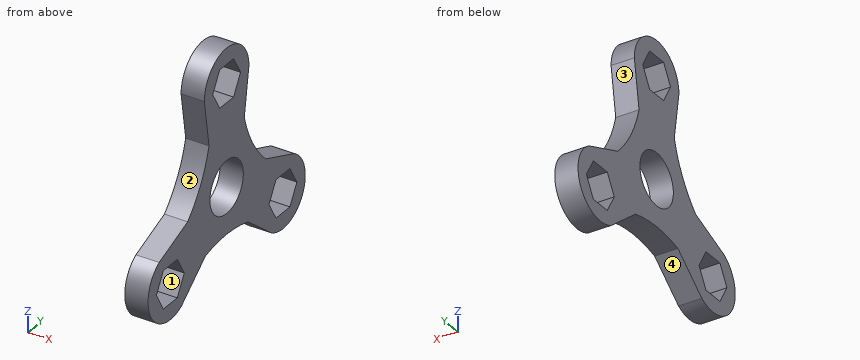
```python
from build123d import *

# Parameters (mm, degrees)
F0_R     = 9
F1_DEPTH = 8


with BuildPart() as f1:
    # F0 (on Right) → F1 (new body)
    with BuildSketch(Plane.YZ):
        with BuildLine():
            Line((9.482996, 18.707991), (12, 35))
            ThreePointArc((12, 35), (0, 47), (-12, 35))
            Line((-12, 35), (-9.482996, 18.707991))
            ThreePointArc((-9.482996, 18.707991), (-13.851316, 7.997061), (-20.943094, -1.14148))
            Line((-20.943094, -1.14148), (-36.310889, -7.107695))
            ThreePointArc((-36.310889, -7.107695), (-40.703194, -23.5), (-24.310889, -27.892305))
            Line((-24.310889, -27.892305), (-11.460098, -17.566512))
            ThreePointArc((-11.460098, -17.566512), (0, -15.994123), (11.460098, -17.566512))
            Line((11.460098, -17.566512), (24.310889, -27.892305))
            ThreePointArc((24.310889, -27.892305), (40.703194, -23.5), (36.310889, -7.107695))
            Line((36.310889, -7.107695), (20.943094, -1.14148))
            ThreePointArc((20.943094, -1.14148), (13.851316, 7.997061), (9.482996, 18.707991))
        make_face()
        Polygon((-26.558112, -11), (-22.805336, -17.5), (-26.558112, -24), (-34.063666, -24), (-37.816443, -17.5), (-34.063666, -11), align=None, mode=Mode.SUBTRACT)
        Polygon((22.805336, -17.5), (26.558112, -11), (34.063666, -11), (37.816443, -17.5), (34.063666, -24), (26.558112, -24), align=None, mode=Mode.SUBTRACT)
        Circle(F0_R, mode=Mode.SUBTRACT)
        Polygon((7.505553, 35), (3.752777, 28.5), (-3.752777, 28.5), (-7.505553, 35), (-3.752777, 41.5), (3.752777, 41.5), align=None, mode=Mode.SUBTRACT)
    extrude(amount=F1_DEPTH)


solid = f1.part
```
Work out the finished part from the listing and answer in its coordinate system (mm). Face numbers are marked on the shaded views. A direction names the side the tool comes from. Give positions to 0.01 mm unless a question says otherwise; leave off trailing zeros. Loops run counter-clockwise (first coordinate to the right, second up) from the corner with the lowest first, then second, coordinate; pieces in that order, holes last. Notation, with made-up numbers: (-13.5, -28) - (28.5, -28) arc R19 ccw to (28.5, -5) - close; hole circle Ø7 at (8, 40). An arc over 180 degrees is marked (long way). Use CSV: the item, a comma, the result in double quotes. Start each with the question number.
(1) Find section B-B, the plane x = 4.5. Count the separate pieces of the cut face and the enclosed holes in it, plus the area to 3 significant figures.
(2) A tool of negligible diameter and unlimited length cuts with its end or side. For the marked faces 1, 2, 3 and 4, from which of +Z, -Z, +X, -X, +Y, -Y can it reach the whole face along a straight path? Write none if from no direction.
(3) Find section D-D, the plane z = 36. Determine the outline of the cut face in (x, y).
(4) Each of these flat-tipped pins is pushed along its axis until it touches: pin 1 (4 mm diameter, centred on x = 3.5, y = -30, fed in from +Z); pin 2 (4 mm diameter, centred on x = 2.5, y = 30.5, fed in from +Z); pin 3 (2.5 mm diameter, centred on x = 4.5, y = -32, fed in from -Z). Where does it stop, or does it pass through?
(5) Find section C-C, the plane z = -22.5. Determine the outline of the cut face in (x, y), plus the area to 3 significant figures.
(6) Find section A-A, the plane y = 0. Determine the outline of the cut face in (x, z).
(7) Find the intervals of material crossed by L1, parallel to Z at x = 2, y = 0; L2, parallel to Y at x = 4.5, z = -14.5; L3, parallel to Z at x = 3.25, y = -5, in increasing order.
Results found:
1,separate pieces,"1"
1,enclosed holes,"4"
1,area,"2,100 mm^2"
2,face 1,"+X, -X"
2,face 2,"+X, -X, -Y"
2,face 3,"+X, -X, +Y"
2,face 4,"-Z, +X, -X"
3,outline,"(0, -11.96) - (8, -11.96) - (8, -6.93) - (0, -6.93) - close; (0, 6.93) - (8, 6.93) - (8, 11.96) - (0, 11.96) - close"
4,pin 1,"z = -3.88"
4,pin 2,"z = -4.08"
4,pin 3,"z = -29.49"
5,outline,"(0, -41.22) - (8, -41.22) - (8, -34.93) - (0, -34.93) - close; (0, -25.69) - (8, -25.69) - (8, -17.6) - (0, -17.6) - close; (0, 17.6) - (8, 17.6) - (8, 25.69) - (0, 25.69) - close; (0, 34.93) - (8, 34.93) - (8, 41.22) - (0, 41.22) - close"
5,area,"230 mm^2"
6,outline,"(0, -15.99) - (8, -15.99) - (8, -9) - (0, -9) - close; (0, 9) - (8, 9) - (8, 28.5) - (0, 28.5) - close; (0, 41.5) - (8, 41.5) - (8, 47) - (0, 47) - close"
7,L1,"-15.99 to -9, 9 to 28.5, 41.5 to 47"
7,L2,"-41.93 to -36.08, -24.54 to 24.54, 36.08 to 41.93"
7,L3,"-16.29 to -7.48, 7.48 to 30.66, 39.34 to 45.91"
